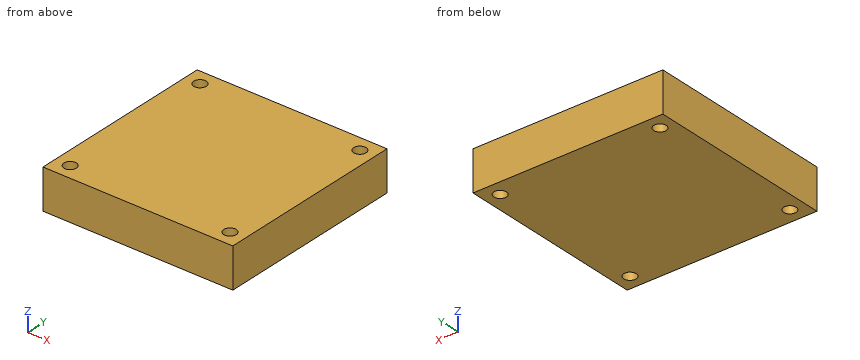
```python
from build123d import *

# Parameters (mm, degrees)
SKETCH1_W               = 38
SKETCH1_H               = 38
BOSS_EXTRUDE1_DEPTH     = 4
SKETCH2_R               = 1.25
CUT_EXTRUDE1_DEPTH      = 9
MIRROR2_COPY_1_SKETCH_R = 1.25
MIRROR2_COPY_1_DEPTH    = 9


with BuildPart() as part:
    # Sketch1 → Boss-Extrude1 (new body, symmetric)
    with BuildSketch(Plane.XY):
        Rectangle(SKETCH1_W, SKETCH1_H)
    extrude(amount=BOSS_EXTRUDE1_DEPTH, both=True)

    # Sketch2 → Cut-Extrude1 (cut, through all)
    with BuildSketch(Plane.XY.offset(4)):
        with Locations((-16, 16)):
            Circle(SKETCH2_R)
    cut_extrude1 = extrude(amount=-CUT_EXTRUDE1_DEPTH, mode=Mode.SUBTRACT)

    # Mirror1: Cut-Extrude1 across plane
    add(cut_extrude1.mirror(Plane.ZX), mode=Mode.SUBTRACT)

    # Mirror2: Cut-Extrude1 across plane
    add(cut_extrude1.mirror(Plane(origin=(0, 0, 0), x_dir=(0, 0, 1), z_dir=(1, 0, 0))), mode=Mode.SUBTRACT)

    # Mirror2 copy 1 sketch → Mirror2 copy 1 (cut, through all)
    with BuildSketch(Plane(origin=(0, 0, 4), x_dir=(-1, 0, 0), z_dir=(0, 0, 1))):
        with Locations((-16, 16)):
            Circle(MIRROR2_COPY_1_SKETCH_R)
    extrude(amount=-MIRROR2_COPY_1_DEPTH, mode=Mode.SUBTRACT)


solid = part.part
```
Model file for the job. Use its own axes, mm. Coordinates: 2 decimals unless noted, no trailing zeros. Write each loop counter-clockwise with the first axis right and the second up, starting at its lowest first coordinate (ties: lowest second). Pieces come first, ordered by that corner, then holes. Notation, with made-up numbers: (-2, 5.5) - (15, 5.5) arc R30 ccw to (15, 31.5) - close; hole circle Ø9 at (47, 79.5). An arc over 180 degrees is marked (long way). Use a Markdown table: item, result. Add a question column.
Item 1: Drill centre lines: line 1 along Y through (x, z) = (16, 2.25); line 2 along X through (y, z) = (16.5, -0.75). Where is each one in solid material? Low to high.
Item 2: Band-saw the part on A-A, the plane y = 16. Write the cut outline in (x, z), and give its area (3 significant figures).
Item 3: Drop a flat-ended pin along its axis: pin 1 (2 mm diameter, centred on x = -16, y = 16, fed in from +Z). Give the stop position or say it passes through.
A:
| question | item | result |
|---|---|---|
| 1 | line 1 | y = -19 to -17.25, -14.75 to 14.75, 17.25 to 19 |
| 1 | line 2 | x = -19 to -17.15, -14.85 to 14.85, 17.15 to 19 |
| 2 | outline | (-19, -4) - (-17.25, -4) - (-17.25, 4) - (-19, 4) - close; (-14.75, -4) - (14.75, -4) - (14.75, 4) - (-14.75, 4) - close; (17.25, -4) - (19, -4) - (19, 4) - (17.25, 4) - close |
| 2 | area | 264 mm² |
| 3 | pin 1 | passes through |
